```python
from build123d import *

# Parameters (mm, degrees)
SKETCH1_W                                       = 119.634
SKETCH1_H                                       = 95.25
BOSS_EXTRUDE1_DEPTH                             = 3.81
FILLET1_R                                       = 3.175
BOSS_EXTRUDE2_DEPTH                             = 2.032
CSK_FOR_M3_FLAT_HEAD_MACHINE_SCREW1_D           = 3.4
CSK_FOR_M3_FLAT_HEAD_MACHINE_SCREW1_DEPTH       = 25.4
CSK_FOR_M3_FLAT_HEAD_MACHINE_SCREW1_CSINK_D     = 6.3
CSK_FOR_M3_FLAT_HEAD_MACHINE_SCREW1_CSINK_ANGLE = 90
CSK_FOR_M3_FLAT_HEAD_MACHINE_SCREW1_TIP         = 1.021463052


with BuildPart() as part:
    # Sketch1 → Boss-Extrude1 (new body)
    with BuildSketch(Plane(origin=(0, 0, 0), x_dir=(1, 0, 0), z_dir=(0, 1, 0))):
        with Locations((59.817, 47.625)):
            Rectangle(SKETCH1_W, SKETCH1_H)
    extrude(amount=BOSS_EXTRUDE1_DEPTH)

    # Fillet1
    fillet1_edges = [part.edges().sort_by_distance(p)[0] for p in [
        (59.817, 0, -95.25),
        (119.634, 0, -47.625),
        (59.817, 0, 0),
        (0, 0, -47.625),
        (0, 1.905, -95.25),
        (119.634, 1.905, -95.25),
        (119.634, 1.905, 0),
        (0, 1.905, 0),
    ]]
    fillet(fillet1_edges, radius=FILLET1_R)

    # Sketch2 → Boss-Extrude2 (add)
    with BuildSketch(Plane(origin=(0, 3.81, 0), x_dir=(1, 0, 0), z_dir=(0, 1, 0))):
        with BuildLine():
            Line((9.076232935, 92.71), (110.557767065, 92.71))
            ThreePointArc((110.557767065, 92.71), (111.500790054, 86.90936796), (117.348, 86.320504417))
            Line((117.348, 86.320504417), (117.348, 8.929495583))
            ThreePointArc((117.348, 8.929495583), (111.500790054, 8.34063204), (110.557767065, 2.54))
            Line((110.557767065, 2.54), (9.076232935, 2.54))
            ThreePointArc((9.076232935, 2.54), (8.133209946, 8.34063204), (2.286, 8.929495583))
            Line((2.286, 8.929495583), (2.286, 86.320504417))
            ThreePointArc((2.286, 86.320504417), (8.133209946, 86.90936796), (9.076232935, 92.71))
        make_face()
        with BuildLine():
            Line((11.679294682, 90.678), (107.954705318, 90.678))
            ThreePointArc((107.954705318, 90.678), (110.049437362, 85.485554332), (115.316, 83.584840695))
            Line((115.316, 83.584840695), (115.316, 11.665159305))
            ThreePointArc((115.316, 11.665159305), (110.049437362, 9.764445668), (107.954705318, 4.572))
            Line((107.954705318, 4.572), (11.679294682, 4.572))
            ThreePointArc((11.679294682, 4.572), (9.584562638, 9.764445668), (4.318, 11.665159305))
            Line((4.318, 11.665159305), (4.318, 83.584840695))
            ThreePointArc((4.318, 83.584840695), (9.584562638, 85.485554332), (11.679294682, 90.678))
        make_face(mode=Mode.SUBTRACT)
    extrude(amount=BOSS_EXTRUDE2_DEPTH)

    # CSK for M3 Flat Head Machine Screw1
    with Locations(Plane(origin=(0, 0, 0), x_dir=(-1, 0, 0), z_dir=(0, -1, 0))):
        with Locations((-114.427, 5.207), (-5.207, 5.207), (-5.207, 90.043), (-114.427, 90.043)):
            CounterSinkHole(CSK_FOR_M3_FLAT_HEAD_MACHINE_SCREW1_D / 2, CSK_FOR_M3_FLAT_HEAD_MACHINE_SCREW1_CSINK_D / 2, depth=CSK_FOR_M3_FLAT_HEAD_MACHINE_SCREW1_DEPTH, counter_sink_angle=CSK_FOR_M3_FLAT_HEAD_MACHINE_SCREW1_CSINK_ANGLE)
            with Locations((0, 0, -(CSK_FOR_M3_FLAT_HEAD_MACHINE_SCREW1_DEPTH + CSK_FOR_M3_FLAT_HEAD_MACHINE_SCREW1_TIP / 2))):  # 118° drill point
                Cone(0, CSK_FOR_M3_FLAT_HEAD_MACHINE_SCREW1_D / 2, CSK_FOR_M3_FLAT_HEAD_MACHINE_SCREW1_TIP, mode=Mode.SUBTRACT)


solid = part.part
```
Could you check a few things on this model? Use its own coordinates, in mm. A direction names the side the tool comes from. Round coordinates to 2 decimals unless told otherwise and drop trailing zeros. Order: outer loops, then holes, each group sorted by start corner. A loop starts at its lowest first (then second) coordinate and runs counter-clockwise, first axis right, second up. Notation, with made-up numbers: M -5.75,55.25 L 9.25,55.25 A20 ccw 9.25,78.25 Z; hole C 81.25,33 d9. An arc over 180 degrees is marked long. One line per question, with ' | ' between items. Start each with the question number.
(1) For P1, Ø2, axis at x = 48.5, y = 4.5, coming from the -Z side; P2, Ø2, axis at y = 5, z = -56, coming from the -X side; P3, Ø2.5, axis at x = 5.207, z = -90.043, coming from the -Y side; P4, Ø1.6, axis at x = 42.5, y = 5, coming from the +Z side, each with a flat end and sliding along its axis, tell me the tip position at first contact or that it passes through.
(2) Suppose I cut it at A-A on x = 20. List the corners of the cut face in (y, z) for me (3 decimals).
(3) Thinking about a two-plate mould opening in Z: for faces 3 (the face through (60.61, 0.95, -0.91)), 4 (the face through (116, 2.65, -4.56)), 5 (the face through (59, 0, -48)), which applies, +Z half, -Z half, draft (parallel to the pull), parting line (faces both ways), or undercut?
(4) Please list where these lines run through material, in increasing order: line 1 along Z through (x, y) = (92, 5); line 2 along X through (y, z) = (5.5, -19.5); line 3 along Y through (x, z) = (114, -43).
(5) For faces 1 (the face through (116.05, 2.65, -90.55)), 2 (the face through (8.07, 4.81, -86.85)), which set-ups out of +Z, -Z, +X, -X, +Y, -Y let a thin tool reach every point of the face, with its end or its side?
(6) Suppose I cut it at B-B on z = -41. List the corners of the cut face in (x, y) for me (3 decimals).
Geometry results:
1) P1: z = -95.25 | P2: x = 2.29 | P3: through | P4: z = -2.54
2) outline: M 0,-92.075 A3.175 ccw 3.175,-95.25 L 3.81,-95.25 L 3.81,-92.71 L 5.842,-92.71 L 5.842,-90.678 L 3.81,-90.678 L 3.81,-4.572 L 5.842,-4.572 L 5.842,-2.54 L 3.81,-2.54 L 3.81,0 L 3.175,0 A3.175 ccw 0,-3.175 Z
3) face 3: +Z half | face 4: undercut | face 5: draft
4) line 1: -92.71 to -90.68, -4.57 to -2.54 | line 2: 2.29 to 4.32, 115.32 to 117.35 | line 3: 0 to 3.81
5) face 1: +Y, -Y | face 2: +Y
6) outline: M 0,3.175 A3.175 ccw 3.175,0 L 116.459,0 A3.175 ccw 119.634,3.175 L 119.634,3.81 L 117.348,3.81 L 117.348,5.842 L 115.316,5.842 L 115.316,3.81 L 4.318,3.81 L 4.318,5.842 L 2.286,5.842 L 2.286,3.81 L 0,3.81 Z
